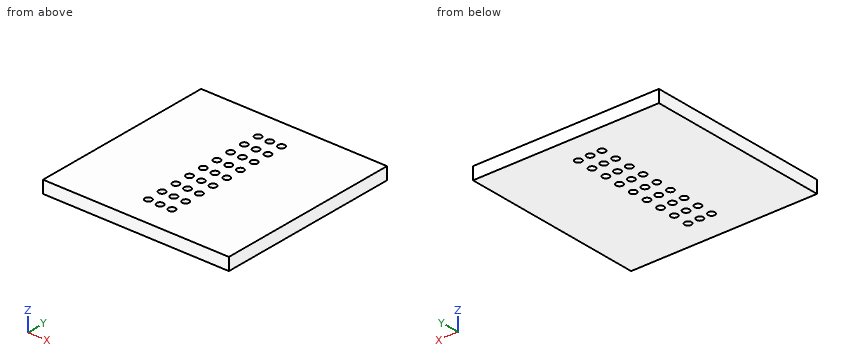
from build123d import *

# Parameters (mm, degrees)
ESQUISSE1_W            = 30
ESQUISSE1_H            = 30
BASE_PLATE_DEPTH       = 2
SKETCH_PERFORATIONS_R  = 0.55
CUT_PERFORATIONS_DEPTH = 10


with BuildPart() as part:
    # Esquisse1 → Base_Plate (new body)
    with BuildSketch(Plane.XY):
        Rectangle(ESQUISSE1_W, ESQUISSE1_H)
    extrude(amount=BASE_PLATE_DEPTH)

    # Sketch_Perforations → Cut_Perforations (cut)
    with BuildSketch(Plane.XY.offset(2)):
        with Locations((-1.9, -10.4)):
            Circle(SKETCH_PERFORATIONS_R)
        with Locations((-1.9, -7.8)):
            Circle(SKETCH_PERFORATIONS_R)
        with Locations((-1.9, -5.2)):
            Circle(SKETCH_PERFORATIONS_R)
        with Locations((-1.9, -2.6)):
            Circle(SKETCH_PERFORATIONS_R)
        with Locations((-1.9, 0)):
            Circle(SKETCH_PERFORATIONS_R)
        with Locations((-1.9, 2.6)):
            Circle(SKETCH_PERFORATIONS_R)
        with Locations((-1.9, 5.2)):
            Circle(SKETCH_PERFORATIONS_R)
        with Locations((-1.9, 7.8)):
            Circle(SKETCH_PERFORATIONS_R)
        with Locations((-1.9, 10.4)):
            Circle(SKETCH_PERFORATIONS_R)
        with Locations((0, -10.4)):
            Circle(SKETCH_PERFORATIONS_R)
        with Locations((0, -7.8)):
            Circle(SKETCH_PERFORATIONS_R)
        with Locations((0, -5.2)):
            Circle(SKETCH_PERFORATIONS_R)
        with Locations((0, -2.6)):
            Circle(SKETCH_PERFORATIONS_R)
        Circle(SKETCH_PERFORATIONS_R)
        with Locations((0, 2.6)):
            Circle(SKETCH_PERFORATIONS_R)
        with Locations((0, 5.2)):
            Circle(SKETCH_PERFORATIONS_R)
        with Locations((0, 7.8)):
            Circle(SKETCH_PERFORATIONS_R)
        with Locations((0, 10.4)):
            Circle(SKETCH_PERFORATIONS_R)
        with Locations((1.9, -10.4)):
            Circle(SKETCH_PERFORATIONS_R)
        with Locations((1.9, -7.8)):
            Circle(SKETCH_PERFORATIONS_R)
        with Locations((1.9, -5.2)):
            Circle(SKETCH_PERFORATIONS_R)
        with Locations((1.9, -2.6)):
            Circle(SKETCH_PERFORATIONS_R)
        with Locations((1.9, 0)):
            Circle(SKETCH_PERFORATIONS_R)
        with Locations((1.9, 2.6)):
            Circle(SKETCH_PERFORATIONS_R)
        with Locations((1.9, 5.2)):
            Circle(SKETCH_PERFORATIONS_R)
        with Locations((1.9, 7.8)):
            Circle(SKETCH_PERFORATIONS_R)
        with Locations((1.9, 10.4)):
            Circle(SKETCH_PERFORATIONS_R)
    extrude(amount=-CUT_PERFORATIONS_DEPTH, mode=Mode.SUBTRACT)


solid = part.part
Geometry check sheet. Reference: the model listing, model coordinates, mm. Round coordinates to 2 decimals unless told otherwise and drop trailing zeros. Write each loop counter-clockwise with the first axis right and the second up, starting at its lowest first coordinate (ties: lowest second). Pieces come first, ordered by that corner, then holes.
Item 1: Section check B-B (y = 5.2). Record the boundary of the cut face in (x, z), plus the area to 3 significant figures.
Determined:
outline: (-15, 0) - (-2.45, 0) - (-2.45, 2) - (-15, 2) - close; (-1.35, 0) - (-0.55, 0) - (-0.55, 2) - (-1.35, 2) - close; (0.55, 0) - (1.35, 0) - (1.35, 2) - (0.55, 2) - close; (2.45, 0) - (15, 0) - (15, 2) - (2.45, 2) - close
area: 53.4 mm2
Item 2: Go/stop test with a flat-tipped pin: pin 1 Ø4 at (x, y) = (-9, -7.5) entering from -Z. Record where the tip stops, or that it passes through.
Determined:
pin 1: stops at z = 0
Item 3: Section check A-A (z = 1.65). Give the number of separate pieces and of enclosed holes in the cut face, plus the area to 3 significant figures.
Determined:
separate pieces: 1
enclosed holes: 27
area: 874 mm2
Item 4: Material ranges on line 1 along X through (y, z) = (3, 0.5), recorded low to high.
Determined:
line 1: x = -15 to -2.28, -1.52 to -0.38, 0.38 to 1.52, 2.28 to 15
